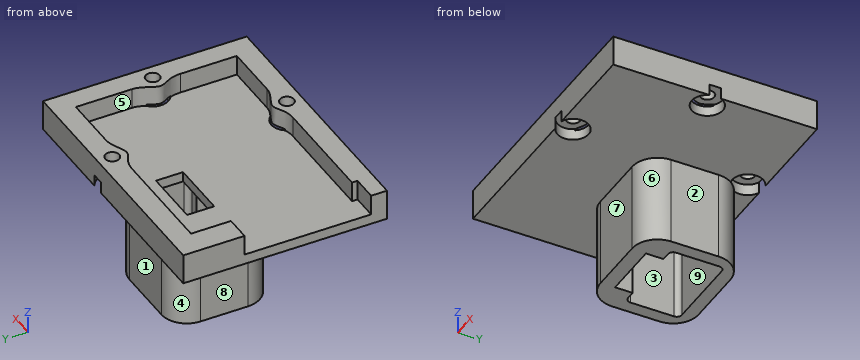
```python
from build123d import *

# Parameters (mm, degrees)
SKETCH11_W          = 20.5
SKETCH11_H          = 16
BOSS_EXTRUDE4_DEPTH = 1.6
SKETCH10_W          = 20.5
SKETCH10_H          = 16
BOSS_EXTRUDE5_DEPTH = 0.8
SKETCH12_R          = 1.225
CUT_EXTRUDE1_DEPTH  = 0.9
SKETCH13_R          = 0.55
CUT_EXTRUDE2_DEPTH  = 1.5
SKETCH14_W          = 4.55
SKETCH14_H          = 2.13
CUT_EXTRUDE3_DEPTH  = 0.8
SKETCH17_W          = 1.985999923
SKETCH17_H          = 9.940122219
CUT_EXTRUDE5_DEPTH  = 1.6
SKETCH18_W          = 8.635
SKETCH18_H          = 7.722
SKETCH18_W_2        = 6.635
SKETCH18_H_2        = 4.222
BOSS_EXTRUDE6_DEPTH = 7
FILLET2_R           = 0.4
FILLET3_R           = 2
SKETCH19_W          = 4.5
SKETCH19_H          = 1.38
CUT_EXTRUDE6_DEPTH  = 7
SKETCH21_W          = 4.5
SKETCH21_H          = 0.8
CUT_EXTRUDE7_DEPTH  = 5.41


with BuildPart() as part:
    # Sketch11 → Boss-Extrude4 (new body)
    with BuildSketch(Plane.XY):
        with Locations((-1.95, 0)):
            Rectangle(SKETCH11_W, SKETCH11_H)
        with BuildLine():
            Line((6.622999053, 6.323000154), (2.19427083, 6.323000154))
            add(Edge.make_bspline(
                [(2.19427083, 6.323000154), (1.446811282, 6.323000154), (0.126304944, 5.123000154), (-0.499421171, 6.323000154), (-1.59427083, 6.323000154)],
                knots=[0, 0, 0, 0, 0.5, 1, 1, 1, 1], degree=3))
            Line((-1.59427083, 6.323000154), (-10.214000077, 6.323000154))
            Line((-10.214000077, 6.323000154), (-10.214000077, -6.323000154))
            Line((-10.214000077, -6.323000154), (-1.59427083, -6.323000154))
            add(Edge.make_bspline(
                [(2.19427083, -6.323000154), (1.446811282, -6.323000154), (0.126304944, -5.123000154), (-0.499421171, -6.323000154), (-1.59427083, -6.323000154)],
                knots=[0, 0, 0, 0, 0.5, 1, 1, 1, 1], degree=3))
            Line((2.19427083, -6.323000154), (6.622999053, -6.323000154))
            Line((6.622999053, -6.323000154), (6.622999053, -1.894271742))
            add(Edge.make_bspline(
                [(6.622999053, 1.894271742), (6.622999053, 1.146811937), (5.422999053, -0.173695015), (6.622999053, -0.799421908), (6.622999053, -1.894271742)],
                knots=[0, 0, 0, 0, 0.5, 1, 1, 1, 1], degree=3))
            Line((6.622999053, 1.894271742), (6.622999053, 6.323000154))
        make_face(mode=Mode.SUBTRACT)
    extrude(amount=BOSS_EXTRUDE4_DEPTH)

    # Sketch10 → Boss-Extrude5 (add)
    with BuildSketch(Plane.XY):
        with Locations((-1.95, 0)):
            Rectangle(SKETCH10_W, SKETCH10_H)
    extrude(amount=-BOSS_EXTRUDE5_DEPTH)

    # Sketch12 → Cut-Extrude1 (cut)
    with BuildSketch(Plane(origin=(0, 0, -0.8), x_dir=(-1, 0, 0), z_dir=(0, 0, -1))):
        with Locations((-0.3, 6.857999949)):
            Circle(SKETCH12_R)
        with Locations((-7.157999783, 0)):
            Circle(SKETCH12_R)
        with Locations((-0.3, -6.857999949)):
            Circle(SKETCH12_R)
    extrude(amount=-CUT_EXTRUDE1_DEPTH, mode=Mode.SUBTRACT)

    # Sketch13 → Cut-Extrude2 (cut)
    with BuildSketch(Plane(origin=(0, 0, 0.1), x_dir=(-1, 0, 0), z_dir=(0, 0, -1))):
        with Locations((-0.3, 6.857999949)):
            Circle(SKETCH13_R)
        with Locations((-7.157999783, 0)):
            Circle(SKETCH13_R)
        with Locations((-0.3, -6.857999949)):
            Circle(SKETCH13_R)
    extrude(amount=-CUT_EXTRUDE2_DEPTH, mode=Mode.SUBTRACT)

    # Sketch14 → Cut-Extrude3 (cut)
    with BuildSketch(Plane(origin=(0, 0, -0.8), x_dir=(-1, 0, 0), z_dir=(0, 0, -1))):
        with Locations((3.953000077, 3.426999846)):
            Rectangle(SKETCH14_W, SKETCH14_H)
    extrude(amount=-CUT_EXTRUDE3_DEPTH, mode=Mode.SUBTRACT)

    # Sketch17 → Cut-Extrude5 (cut)
    with BuildSketch(Plane.XY.offset(1.6)):
        with Locations((-11.207000039, -1.784681503)):
            Rectangle(SKETCH17_W, SKETCH17_H)
    extrude(amount=-CUT_EXTRUDE5_DEPTH, mode=Mode.SUBTRACT)

    # Sketch18 → Boss-Extrude6 (add)
    with BuildSketch(Plane(origin=(0, 0, -0.8), x_dir=(-1, 0, 0), z_dir=(0, 0, -1))):
        with Locations((3.953000077, 2.676999846)):
            Rectangle(SKETCH18_W, SKETCH18_H)
        with Locations((3.953000077, 3.426999846)):
            Rectangle(SKETCH18_W_2, SKETCH18_H_2, mode=Mode.SUBTRACT)
    extrude(amount=BOSS_EXTRUDE6_DEPTH)

    # Fillet2
    fillet2_edges = [part.edges().sort_by_distance(p)[0] for p in [
        (-0.635500077, 5.537999846, -4.3),
        (-0.635500077, 1.315999846, -4.3),
        (-7.270500077, 1.315999846, -4.3),
        (-7.270500077, 5.537999846, -4.3),
    ]]
    fillet(fillet2_edges, radius=FILLET2_R)

    # Fillet3
    # the kernel refuses this fillet: 2 mm, written as the material it takes off along each edge
    with BuildSketch(Plane(origin=(-8.270500077, 6.537999846, -0.8), x_dir=(0, -1, 0), z_dir=(0, 0, -1)), Plane(origin=(0.364499923, -1.184000154, -0.8), x_dir=(0, 1, 0), z_dir=(0, 0, -1)), Plane(origin=(-8.270500077, -1.184000154, -0.8), x_dir=(1, 0, 0), z_dir=(0, 0, -1))) as fillet3_piece_1:
        with BuildLine():
            CenterArc((FILLET3_R, -FILLET3_R), FILLET3_R, 90, 90)
            Line((0, -FILLET3_R), (0, 0))
            Line((0, 0), (FILLET3_R, 0))
        make_face()
    extrude(amount=12, mode=Mode.SUBTRACT)
    with BuildSketch(Plane(origin=(0.364499923, 6.537999846, -0.8), x_dir=(0, -1, 0), z_dir=(0, 0, -1))) as fillet3_piece_2:
        with BuildLine():
            CenterArc((FILLET3_R, FILLET3_R), FILLET3_R, 180, 90)
            Line((0, FILLET3_R), (0, 0))
            Line((0, 0), (FILLET3_R, 0))
        make_face()
    extrude(amount=12, mode=Mode.SUBTRACT)

    # Sketch19 → Cut-Extrude6 (cut)
    with BuildSketch(Plane(origin=(0, 0, -7.8), x_dir=(-1, 0, 0), z_dir=(0, 0, -1))):
        with Locations((3.953000077, 0.625999846)):
            Rectangle(SKETCH19_W, SKETCH19_H)
    extrude(amount=-CUT_EXTRUDE6_DEPTH, mode=Mode.SUBTRACT)

    # Sketch21 → Cut-Extrude7 (cut)
    with BuildSketch(Plane(origin=(0, 0, -6.21), x_dir=(-1, 0, 0), z_dir=(0, 0, -1))):
        with Locations((3.953000077, -0.464000154)):
            Rectangle(SKETCH21_W, SKETCH21_H)
    extrude(amount=-CUT_EXTRUDE7_DEPTH, mode=Mode.SUBTRACT)


solid = part.part
```
CAD build for the part. Positions are in the model's coordinates, mm. Face numbers are marked on the shaded views. A direction names the side the tool comes from. Round coordinates to 2 decimals unless told otherwise and drop trailing zeros. Order: outer loops, then holes, each group sorted by start corner. A loop starts at its lowest first (then second) coordinate and runs counter-clockwise, first axis right, second up. Notation, with made-up numbers: (27.25, 75.25) - (68.25, 75.25) arc R14 cw to (68.25, 102.25) - close; hole circle Ø3 at (57, -13.5). An arc over 180 degrees is marked (long way). Use CSV: the item, a comma, the result in double quotes. Start each with the question number.
1) Two-plate mould, pull along X, no slides. Class the marked faces 1, 2, 3 and 4: pulls with the +X half, pulls with the -X half, needs draft (parallel to the pull), parting line crosses it, or undercut.
2) Pin check, flat tips, straight feed: pin 1 Ø3 at (y, z) = (3, -6) entering from -X; pin 2 Ø1.5 at (y, z) = (-3.5, -3) entering from -X; pin 3 Ø2 at (x, y) = (7.158, 0) entering from -Z; pin 4 Ø5 at (x, z) = (-3, -5) entering from +Y. Stop position of each tip, or through.
3) Saw through at B-B (x = -4.75). List the corners of the cut face in (y, z).
4) Saw through at D-D (z = -7). List the corners of the cut face in (x, y).
5) Tool access for the marked faces 5, 6, 7, 8 and 9: list every direction of +Z, -Z, +X, -X, +Y, -Y with a clear straight run to the whole face (end or side of a thin tool).
6) Saw through at A-A (z = -5). List the corners of the cut face in (x, y), and give its area (3 significant figures).
7) Wall check: L1, parallel to X at y = 1, z = -5; L2, parallel to Y at x = -6, z = -6.5; L3, parallel to X at y = 4.5, z = -6. Give the ranges that are in metal, low to high. Write a range as [from, to].
8) Saw through at C-C (y = -5.25). List the corners of the cut face in (x, z), and give its area (3 significant figures).
Values follow:
1,face 1,"needs draft"
1,face 2,"pulls with the +X half"
1,face 3,"undercut"
1,face 4,"pulls with the -X half"
2,pin 1,"stops at x = -8.27"
2,pin 2,"passes through"
2,pin 3,"stops at z = 0.1"
2,pin 4,"stops at y = 6.54"
3,outline,"(-8, -0.8) - (-1.18, -0.8) - (-1.18, -7.8) - (-0.06, -7.8) - (-0.06, -6.21) - (-0.86, -6.21) - (-0.86, -0.8) - (2.36, -0.8) - (2.36, 0) - (-6.32, 0) - (-6.32, 1.6) - (-8, 1.6) - close; (4.49, -0.8) - (5.54, -0.8) - (5.54, -7.8) - (6.54, -7.8) - (6.54, -0.8) - (8, -0.8) - (8, 1.6) - (6.32, 1.6) - (6.32, 0) - (4.49, 0) - close"
4,outline,"(-8.27, 0.82) arc R2 ccw to (-6.27, -1.18) - (-1.64, -1.18) arc R2 ccw to (0.36, 0.82) - (0.36, 4.54) arc R2 ccw to (-1.64, 6.54) - (-6.27, 6.54) arc R2 ccw to (-8.27, 4.54) - close; hole (-7.27, 1.72) arc R0.4 ccw to (-6.87, 1.32) - (-6.2, 1.32) - (-6.2, -0.06) - (-1.7, -0.06) - (-1.7, 1.32) - (-1.04, 1.32) arc R0.4 ccw to (-0.64, 1.72) - (-0.64, 5.14) arc R0.4 ccw to (-1.04, 5.54) - (-6.87, 5.54) arc R0.4 ccw to (-7.27, 5.14) - close"
5,face 5,"+Z"
5,face 6,"-Z, +X, -Y"
5,face 7,"-Z, +X, -X, -Y"
5,face 8,"-Z, -X, +Y, -Y"
5,face 9,"-Z"
6,outline,"(-8.27, 0.82) arc R2 ccw to (-6.27, -1.18) - (-1.64, -1.18) arc R2 ccw to (0.36, 0.82) - (0.36, 4.54) arc R2 ccw to (-1.64, 6.54) - (-6.27, 6.54) arc R2 ccw to (-8.27, 4.54) - close; hole (-7.27, 1.72) arc R0.4 ccw to (-6.87, 1.32) - (-6.2, 1.32) - (-6.2, -0.86) - (-1.7, -0.86) - (-1.7, 1.32) - (-1.04, 1.32) arc R0.4 ccw to (-0.64, 1.72) - (-0.64, 5.14) arc R0.4 ccw to (-1.04, 5.54) - (-6.87, 5.54) arc R0.4 ccw to (-7.27, 5.14) - close"
6,area,"25.6 mm2"
7,L1,"x = [-8.27, -6.2], [-1.7, 0.36]"
7,L2,"y = [-1.18, -0.06], [5.54, 6.54]"
7,L3,"x = [-8.27, -7.27], [-0.64, 0.36]"
8,outline,"(-12.2, -0.8) - (8.3, -0.8) - (8.3, 1.6) - (6.62, 1.6) - (6.62, 0) - (-12.2, 0) - close"
8,area,"19.1 mm2"
